For this review, take the finished solid that the model builds, in its own axes (mm). A direction names the side the tool comes from. Coordinates: 2 decimals unless noted, no trailing zeros. Order: outer loops, then holes, each group sorted by start corner. A loop starts at its lowest first (then second) coordinate and runs counter-clockwise, first axis right, second up. Notation, with made-up numbers: (84.25, -26) -> (130.25, -26) arc R11 cw to (130.25, -9) -> close; hole circle Ø5 at (55, -5.5). An arc over 180 degrees is marked (long way). Write item = value, one per line. Start each with the question number.
1) Consider section A-A on z = 0. Give the boundary of the cut face in (x, y).
2) Machinability: for faces 1 (the face through (-30.62, -12.52, 13.92)), 2 (the face through (-47.7, 25, -3.1)), 3 (the face through (-3.3, -88.01, -14.88)), which of the approach directions +Z, -Z, +X, -X, +Y, -Y give a long, thin tool a straight path to every point of the face, cutting with its end or side? Answer none if there is none.
3) Wall thickness on probe 1 along Y at (x, z) = (1, 9); probe 2 along Y at (x, z) = (-25.5, -7); probe 3 along X at (y, z) = (-3, 0): over which ranges is each line inside the solid? List them lowest first. Write a range as [from, to].
4) Consider section C-C on y = -123. Give the boundary of the cut face in (x, z), and give its area (3 significant figures).
5) Consider section B-B on x = 0. Give the boundary of the cut face in (y, z).
6) Consider section D-D on x = -49. Give the boundary of the cut face in (y, z), and give its area (3 significant figures).
7) Insertion check: pin 1 Ø4 at (y, z) = (-121, -10) entering from +X; pin 2 Ø12 at (y, z) = (-73.5, -6.5) entering from -X; pin 3 Ø5 at (x, y) = (-6.5, -100) entering from -Z. Each pin has a flat end and moves straight along its axis. Give the tip position at first contact, or say it passes through.
from build123d import *

# Parameters (mm, degrees)
F0_R     = 15.24
F1_DEPTH = 152.4
F3_DEPTH = 25.4
F4_R     = 8.05635
F5_DEPTH = 50.8


with BuildPart() as f1:
    # F0 (on Front) → F1 (new body)
    with BuildSketch(Plane.XZ):
        Circle(F0_R)
    extrude(amount=F1_DEPTH)

    # F2 (on Front) → F3 (join)
    with BuildSketch(Plane.XZ):
        with BuildLine():
            Line((-58.810396, -9.067713), (-3.208219, -18.63846))
            ThreePointArc((-3.208219, -18.63846), (18.912558, 0), (-3.208219, 18.63846))
            Line((-3.208219, 18.63846), (-58.810396, 9.067713))
            ThreePointArc((-58.810396, 9.067713), (-66.450643, 0), (-58.810396, -9.067713))
        make_face()
    extrude(amount=F3_DEPTH)

    # F4 (on Front) → F5 (join)
    with BuildSketch(Plane.XZ):
        with Locations((-55.136111, 0)):
            Circle(F4_R)
    extrude(amount=-F5_DEPTH)


solid = f1.part
Answer sheet:
q1.outline = (-66.45, -25.4) -> (-15.24, -25.4) -> (-15.24, -152.4) -> (15.24, -152.4) -> (15.24, -25.4) -> (18.91, -25.4) -> (18.91, 0) -> (-47.08, 0) -> (-47.08, 50.8) -> (-63.19, 50.8) -> (-63.19, 0) -> (-66.45, 0) -> close
q2.face_1 = +Z, -X, +Y, -Y
q2.face_2 = +Y
q2.face_3 = -Y
q3.probe_1 = [-152.4, 0]
q3.probe_2 = [-25.4, 0]
q3.probe_3 = [-66.45, 18.91]
q4.outline = circle Ø30.48 at (0, 0)
q4.area = 730 mm2
q5.outline = (-152.4, -15.24) -> (-25.4, -15.24) -> (-25.4, -18.91) -> (0, -18.91) -> (0, 18.91) -> (-25.4, 18.91) -> (-25.4, 15.24) -> (-152.4, 15.24) -> close
q6.outline = (-25.4, -10.76) -> (0, -10.76) -> (0, -5.22) -> (50.8, -5.22) -> (50.8, 5.22) -> (0, 5.22) -> (0, 10.76) -> (-25.4, 10.76) -> close
q6.area = 1,080 mm2
q7.pin_1 = 12.97
q7.pin_2 = -15.23
q7.pin_3 = -14.71
